Study the drawing (mm; zero at the part's minimum x, y, z) and answer. Round coordinates to 2 decimals unless told otherwise and drop trailing zeros. Write each loop counter-clockwise with the first axis right and the second up, starting at its lowest first coordinate (ties: lowest second). Pieces come first, ordered by that corner, then holes. Notation, with made-up numbers: M -35.5,73 L 15.5,73 A11 cw 15.5,83 Z; hole C 34,40 d11. An arc over 180 degrees is marked long. Write each question's results on one line, items separated by ' | '.
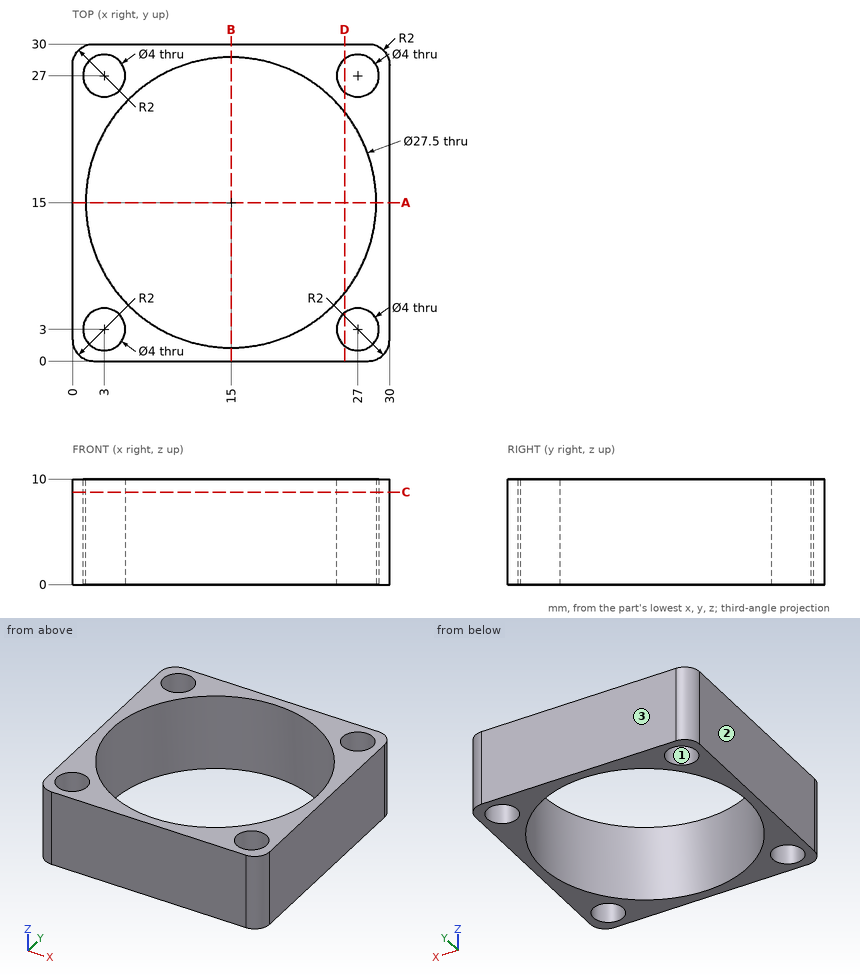
1) This flat-tipped pin is pushed along its axis until it touches: pin 1 (3.5 mm diameter, centred on x = 3, y = 27, fed in from -Z). Where does it stop, or does it pass through?
Return value:
pin 1: through
2) The mould has two halves that part along X. Classify the marked faces 1, 2 and 3: +X half, -X half, draft (parallel to the pull), parting line (faces both ways), or undercut.
Return value:
face 1: undercut | face 2: -X half | face 3: draft
3) Section D-D (x = 25.75) is taken. Determine the outline of the cut face in (y, z).
Return value:
outline: M 0,0 L 1.44,0 L 1.44,10 L 0,10 Z; M 4.56,0 L 6.43,0 L 6.43,10 L 4.56,10 Z; M 23.57,0 L 25.44,0 L 25.44,10 L 23.57,10 Z; M 28.56,0 L 30,0 L 30,10 L 28.56,10 Z
4) Section C-C (z = 8.75) is taken. Determine the outline of the cut face in (x, y).
Return value:
outline: M 0,2 A2 ccw 2,0 L 28,0 A2 ccw 30,2 L 30,28 A2 ccw 28,30 L 2,30 A2 ccw 0,28 Z; hole C 3,3 d4; hole C 3,27 d4; hole C 15,15 d27.5; hole C 27,3 d4; hole C 27,27 d4
5) Find the intervals of material crossed by line 1 (Y direction, x = 4.25, z = 3.5); line 2 (X direction, y = 2.25, z = 2); line 3 (Y direction, x = 27, z = 3.5), in increasing order.
Return value:
line 1: 0 to 1.44, 4.56 to 6.43, 23.57 to 25.44, 28.56 to 30 | line 2: 0 to 1.15, 4.85 to 9.85, 20.15 to 25.15, 28.85 to 30 | line 3: 0 to 1, 5 to 8.29, 21.71 to 25, 29 to 30
6) Section A-A (y = 15) is taken. Determine the outline of the cut face in (x, z), then the cut area to 3 significant figures.
Return value:
outline: M 0,0 L 1.25,0 L 1.25,10 L 0,10 Z; M 28.75,0 L 30,0 L 30,10 L 28.75,10 Z | area: 25.0 mm²
